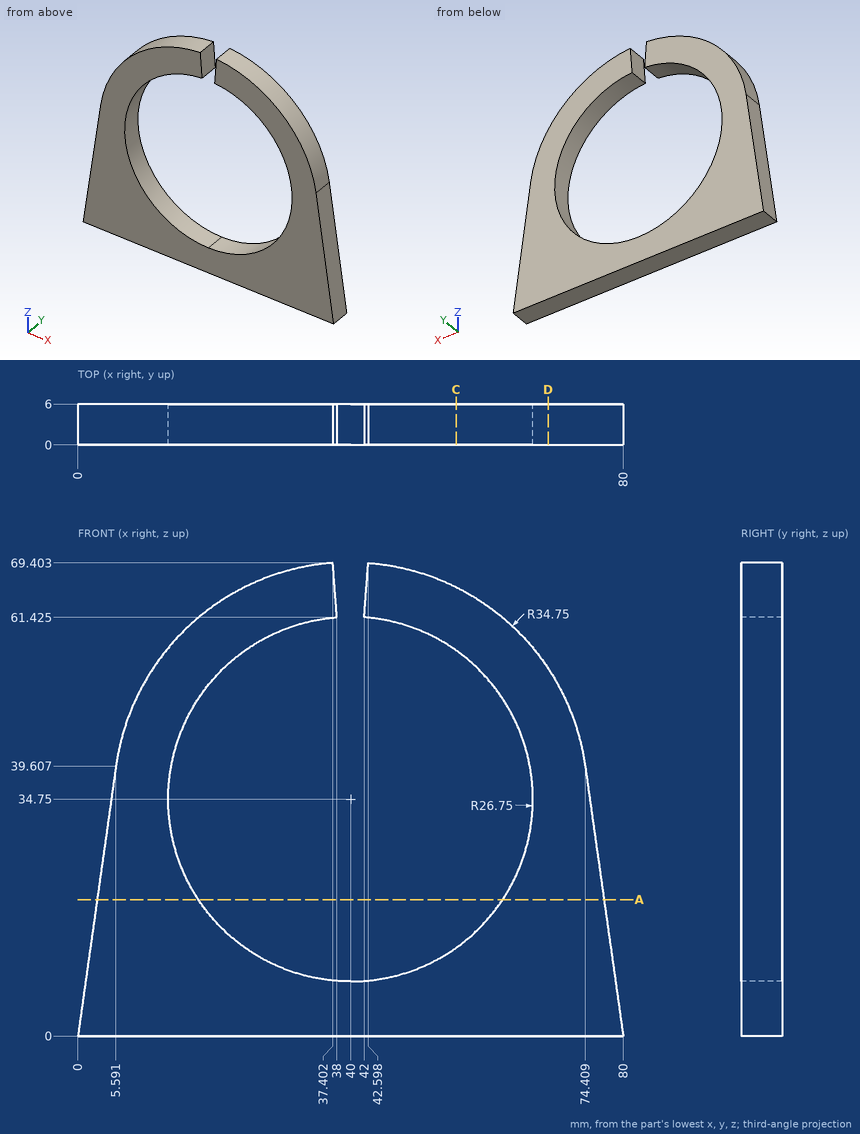
Design review of the part shown in the three views and the two pictorial views. Dimensions are in mm from the part's minimum x, y and z. Round coordinates to 2 decimals unless told otherwise and drop trailing zeros. Loops run counter-clockwise (first coordinate to the right, second up) from the corner with the lowest first, then second, coordinate; pieces in that order, holes last. Notation, with made-up numbers: (13, 35) -> (66, 35) arc R27 cw to (66, 62) -> close; hole circle Ø10 at (8, 69). An arc over 180 degrees is marked (long way). Answer as CSV lines item,"result".
1) Add section A-A on z = 20. Write out the cut boundary in (x, y), plus the area to 3 significant figures.
Geometry results:
outline,"(2.82, 0) -> (17.68, 0) -> (17.68, 6) -> (2.82, 6) -> close; (62.32, 0) -> (77.18, 0) -> (77.18, 6) -> (62.32, 6) -> close"
area,"178 mm²"
2) To check wall thickness, follow line 1 along Z through (x, y) = (26, 3.6) (1 decimal); line 2 along X through (y, z) = (4.65, 58) (1 decimal); line 3 along X through (y, z) = (4.9, 20) (1 decimal). State the ranges of each line that lie inside material, in increasing order. Write a range as from..to.
Geometry results:
line 1,"z = 0..12, 57.5..66.6"
line 2,"x = 14.2..26.8, 53.2..65.8"
line 3,"x = 2.8..17.7, 62.3..77.2"
3) Add section D-D on x = 69. Write out the cut boundary in (y, z).
Geometry results:
outline,"(0, 0) -> (6, 0) -> (6, 53.9) -> (0, 53.9) -> close"
4) Add section C-C on x = 55.5. Write out the cut boundary in (y, z).
Geometry results:
outline,"(0, 0) -> (6, 0) -> (6, 12.95) -> (0, 12.95) -> close; (0, 56.55) -> (6, 56.55) -> (6, 65.85) -> (0, 65.85) -> close"
